Can you work these out from the model? Positions are in its coordinate system, mm. Face numbers are marked on the shaded views. Give positions to 0.01 mm unless a question says otherwise; leave off trailing zeros. Order: outer loops, then holes, each group sorted by start corner. A loop starts at its lowest first (then second) coordinate and runs counter-clockwise, first axis right, second up.
Item 1: If I drill on line 1 along Y through (x, z) = (0, 18); line 2 along X through (y, z) = (-3.5, 29); line 3 along Y through (x, z) = (-5.75, 33), over which ranges is the centre line in solid material (lowest first)?
Item 2: If we mould it in two halves opening along X, with no side actions, what happens to the marked faces 1, 2 and 3? For each: +X half, -X half, draft (parallel to the pull), parting line (faces both ways), or undercut.
Item 3: I'm going to push flat-ended pins straight in: pin 1 Ø4 at (x, z) = (8, 12) entering from -Y; pin 2 Ø2 at (x, z) = (2, 24) entering from +Y; pin 3 Ø3 at (y, z) = (-3, 10) entering from -X. Where does each tip first touch, or does it pass through?
Item 4: I want a section at A-A, the plane z = 33. Write out the boundary of the cut face in (x, y).
Autodesk Inventor part; units mm, degrees
ref_plane "YZ Plane" through (0, 0, 0) normal (1, 0, 0) x (0, 1, 0)
ref_plane "XZ Plane" through (0, 0, 0) normal (0, 1, 0) x (-1, 0, 0)
ref_plane "XY Plane" through (0, 0, 0) normal (0, 0, 1) x (1, 0, 0)
sketch "Sketch1" plane through (0, 0, 50.8) normal (0, 0, 1) x (1, 0, 0)
  circle A0 centre (0, 0) radius 12.7
sketch "Sketch2" plane through (0, 0, 0) normal (0, 1, 0) x (-1, 0, 0)
  line L0 (0, 50.8) -> (-7.62, 50.8)
  line L1 (-7.62, 50.8) -> (-7.62, 3.81)
  arc A0 (-7.62, 3.81) -> (-2.8448, 3.81) centre (-5.2324, 3.81) ccw
  line L2 (-2.8448, 3.81) -> (-2.8448, 9.6774)
  arc A1 (-1.2573, 11.2649) -> (-2.8448, 9.6774) centre (-1.2573, 9.6774) ccw
  line L3 (-1.2573, 11.2649) -> (0, 11.2649)
  line L4 (0, 11.2649) -> (0, 50.8)
  line L5 (0, -10.16) -> (0, 60.96)
extrude "Extrusion1" add sketch "Sketch1" against normal blind 50.8
revolve "Revolution1" cut sketch "Sketch2" angle 360 about axis through (0, 0, -10) along (0, 0, 1)
properties part number "coax_test"
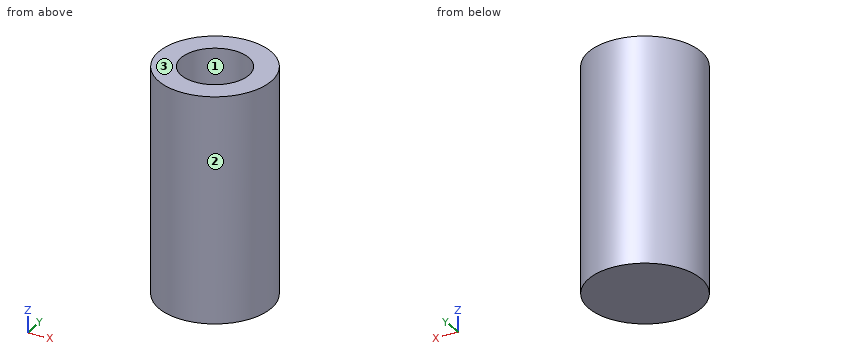
Results list:
1. line 1: y = -12.7 to -7.62, 7.62 to 12.7
1. line 2: x = -12.21 to -6.77, 6.77 to 12.21
1. line 3: y = -11.32 to -5, 5 to 11.32
2. face 1: undercut
2. face 2: parting line
2. face 3: draft
3. pin 1: stops at y = -11.19
3. pin 2: stops at y = 12.66
3. pin 3: stops at x = -12.61
4. outline: circle Ø25.4 at (0, 0); hole circle Ø15.24 at (0, 0)
